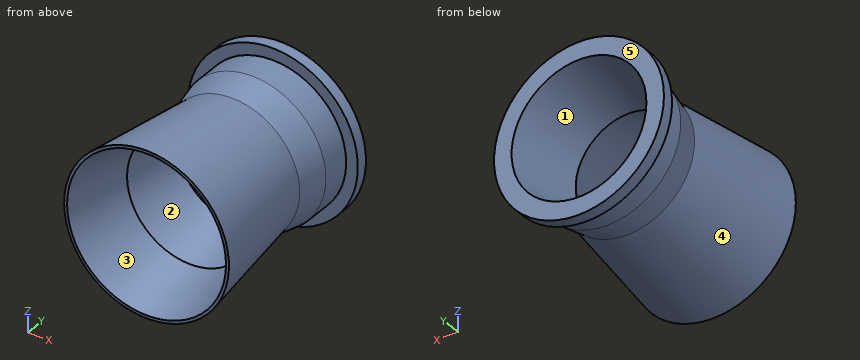
Autodesk Inventor part; units mm, degrees
ref_plane "YZ Plane" through (0, 0, 0) normal (1, 0, 0) x (0, 1, 0)
ref_plane "XZ Plane" through (0, 0, 0) normal (0, 1, 0) x (-1, 0, 0)
ref_plane "XY Plane" through (0, 0, 0) normal (0, 0, 1) x (1, 0, 0)
sketch "Sketch1" plane through (0, 0, 0) normal (0, 0, 1) x (1, 0, 0)
  line L0 (0, 25.4) -> (-28.702, 25.4) construction
  line L1 (0, 25.4) -> (-95.25, 25.4) construction
  line L2 (-95.25, 25.4) -> (-89.1588, 25.4) construction
  line L3 (-89.1588, 25.4) -> (-85.693, 23.7839) construction
  line L4 (-89.1588, 25.4) -> (-89.1588, 21.1626) construction
  line L5 (-89.1588, 0) -> (-95.25, 0)
  line L6 (-28.702, 59.6457) -> (-28.702, -91.9304) construction
  arc A0 (-28.9184, -8.4804) -> (-32.3684, -1.0818) centre (-35.052, -6.8369) ccw
  line L7 (-89.1588, 25.4) -> (-89.1588, 0)
  line L8 (-89.1588, 25.4) -> (-32.3684, -1.0818)
  line L9 (-28.9184, -8.4804) -> (-28.9392, -8.5583)
  line L10 (0, -319.0244) -> (0, 122.7573)
  line L11 (-73.152, 17.9359) -> (-28.702, 17.9359) construction
  line L12 (-89.1588, 0) -> (-92.3338, 0)
  line L13 (11.4547, -6.8369) -> (-136.2084, -6.8369) construction
  line L14 (-57.2892, -89.8271) -> (-74.8171, -155.2422)
  line L15 (-92.3338, -12.7) -> (-73.2838, -12.7)
  line L16 (-73.2838, -12.7) -> (-54.421, -103.6575)
  line L17 (-74.8171, -155.2422) -> (-68.2431, -155.2422)
  line L18 (-92.3338, -25.4) -> (-79.6338, -25.4)
  line L19 (-79.6338, -25.4) -> (-79.6338, -57.15)
  line L20 (-79.6338, -57.15) -> (-72.991, -88.4936)
  line L21 (-92.3338, 0) -> (-92.3338, -25.4)
  line L22 (-86.3902, -25.4) -> (-86.3902, -31.3436)
  line L23 (-86.3902, -31.3436) -> (-92.3338, -31.3436)
  line L24 (-92.3338, -31.3436) -> (-92.3338, -56.7436)
  line L25 (-92.3338, -56.7436) -> (-79.6338, -56.7436)
  line L26 (-73.152, 17.9359) -> (-32.3684, -1.0818)
  line L27 (-73.152, 17.9359) -> (-50.7653, -90.0141)
  line L28 (-50.7653, -90.0141) -> (-28.9184, -8.4804)
  line L29 (-52.4654, -96.3589) -> (-28.9184, -8.4804)
  line L30 (-86.36, -222.8555) -> (-28.9184, -8.4804)
  line L31 (-72.991, -88.4936) -> (-89.535, -222.8555)
  line L32 (-89.535, -222.8555) -> (-86.36, -222.8555)
  point P0 (0, 0)
  point P1 (-95.25, -255.9127)
  point P2 (-88.7095, 22.4389)
  dimension "d0" = 28.702
  dimension "d3" = 25
  dimension "d5" = 25.4
  dimension "d6" = 25.4
  dimension "d8" = 12.7
  dimension "d34" = 15
  dimension "d37" = 44.45
  dimension "d46" = 19.05
  dimension "d47" = 12.7
  dimension "d55" = 12.7
  dimension "d56" = 31.75
  dimension "d58" = 0.25
  dimension "d60" = 12.7
  dimension "d61" = 25.4
  dimension "d62" = 5.9436
  dimension "d63" = 5.9436
  dimension "d64" = 3.175
  dimension "d68" = 107.95
  dimension "d69" = 6.35
  dimension "d70" = 6.35
  dimension "d71" = 3.175
  dimension "d73" = 86.36
  dimension "d74" = 31.75
  dimension "d75" = 6.3448
revolve "Revolution3" add sketch "Sketch1" angle 360 about axis through (0, -10, 0) along (0, 1, 0) contours L15 L16 L14 L17 L30 L32 L31 L20 L19 L18 L21
properties part number "aluminum_carrier" material "Aluminum 6061"
Geometry check sheet. Reference: the model listing, model coordinates, mm. Face numbers are marked on the shaded views. A direction names the side the tool comes from. Coordinates: 2 decimals unless noted, no trailing zeros. Order: outer loops, then holes, each group sorted by start corner. A loop starts at its lowest first (then second) coordinate and runs counter-clockwise, first axis right, second up. Notation, with made-up numbers: (-37.75, 80) - (2.25, 80) arc R10 ccw to (2.25, 89) - close; hole circle Ø4 at (53.25, -31.5). An arc over 180 degrees is marked (long way). One line per item, written item: value.
(1) Depth check by flat-ended pin: pin 1 Ø3 at (y, z) = (-111.5, -66.5) entering from +X; pin 2 Ø2 at (x, y) = (13.5, -84) entering from +Z; pin 3 Ø1.5 at (y, z) = (-147.5, -34.5) entering from -X. Enter the tip coordinate at first touch or a pass-through.
Data:
pin 1: stops at x = 39.07
pin 2: stops at z = 72.98
pin 3: stops at x = -72.83
(2) Access from +Z, -Z, +X, -X, +Y, -Y to the whole of each face (thin tool, end or side, straight path). Record for the marked faces 1 and 2.
Data:
face 1: +Y
face 2: none
(3) Sectioned sample at C-C (y = -45). Enter the section's corners in (x, z), and give its area (3 significant figures).
Data:
outline: circle Ø159.27 at (0, 0); hole circle Ø133.17 at (0, 0)
area: 5,990 mm^2
(4) Release check for a two-part mould opening along Z. For the marked faces 3, 4 and 5 record: +Z half, -Z half, draft (parallel to the pull), parting line (faces both ways), or undercut.
Data:
face 3: undercut
face 4: parting line
face 5: draft
(5) Sectioned sample at D-D (y = -210). Enter the section's corners in (x, z).
Data:
outline: circle Ø175.9 at (0, 0); hole circle Ø165.83 at (0, 0)
(6) Thickness scan on probe 1 along Z at (x, y) = (40.5, -30.5); probe 2 along Z at (x, y) = (-59, -25.5); probe 3 along X at (y, z) = (-56.5, 23.5). Record the ranges inside material, lowest first. Write a range as from..to.
Data:
probe 1: z = -68.57..-56.59, 56.59..68.57
probe 2: z = -53.48..-38.83, 38.83..53.48
probe 3: x = -76.09..-59.74, 59.74..76.09
